Job drawing, mm, ordinate dimensions from the low corner. One solid piece. Give positions to 0.01 mm unless a question says otherwise; leave off trailing zeros. Write each loop counter-clockwise with the first axis right and the second up, starting at its lowest first coordinate (ties: lowest second). Pieces come first, ordered by that corner, then holes. Notation, with made-up numbers: (79.5, -4) - (88.5, -4) arc R23 ccw to (88.5, 23) - close; hole circle Ø4 at (17.25, -37.5). An arc over 180 degrees is marked (long way). Use a Markdown table: item, result. Add a question column.
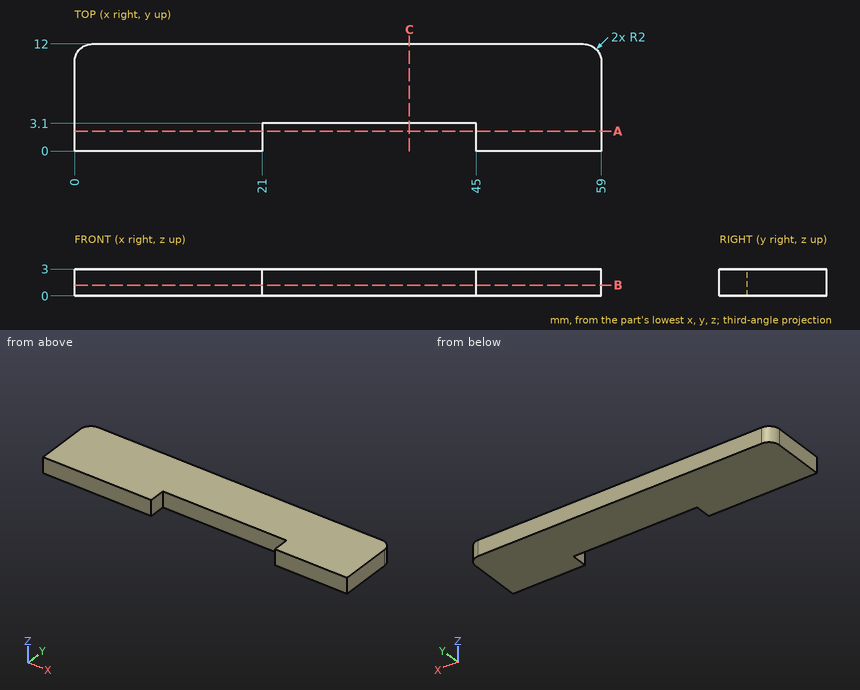
(1) Band-saw the part on A-A (y = 2.25). Write the cut outline in (x, z), then the cut area to 3 significant figures.
(2) Band-saw the part on B-B (z = 1.2). Write the cut outline in (x, y).
(3) Probe probe 1 along X at (y, z) = (0.5, 1.9); probe 2 along Y at (x, z) = (22, 0.5); probe 3 along X at (y, z) = (10.75, 2.6). List the from-to ranges inside material, lowest first. Write a range as [from, to].
(4) Flat gauge pin, fed straight in: pin 1 (4 mm diameter, centred on x = 14.5, y = 1.5, fed in from -Z). Where does the tip first touch, or does it go through?
(5) Band-saw the part on C-C (x = 37.5). Write the cut outline in (y, z).
Model answer:
| question | item | result |
|---|---|---|
| 1 | outline | (0, 0) - (21, 0) - (21, 3) - (0, 3) - close; (45, 0) - (59, 0) - (59, 3) - (45, 3) - close |
| 1 | area | 105 mm^2 |
| 2 | outline | (0, 0) - (21, 0) - (21, 3.1) - (45, 3.1) - (45, 0) - (59, 0) - (59, 10) arc R2 ccw to (57, 12) - (2, 12) arc R2 ccw to (0, 10) - close |
| 3 | probe 1 | x = [0, 21], [45, 59] |
| 3 | probe 2 | y = [3.1, 12] |
| 3 | probe 3 | x = [0.15, 58.85] |
| 4 | pin 1 | stops at z = 0 |
| 5 | outline | (3.1, 0) - (12, 0) - (12, 3) - (3.1, 3) - close |
